Input: part model. Units: mm. Frame: model coordinates. Round coordinates to 2 decimals unless told otherwise and drop trailing zeros. Loops run counter-clockwise (first coordinate to the right, second up) from the corner with the lowest first, then second, coordinate; pieces in that order, holes last. Notation, with made-up numbers: (78, 37.5) - (127, 37.5) arc R5 cw to (127, 44.5) - close; hole circle Ø5 at (-25, 74). An arc over 180 degrees is marked (long way). Use CSV: the item, a comma, the result in double quotes. Start each with the question number.
1. Cut plane A-A (y = 2). Return loops of the section in (x, z), and give its area (3 significant figures).
2. Cut plane B-B (x = 68). Return loops of the section in (y, z).
3. Material intervals for probe 1 along Y at (x, z) = (11.5, 5); probe 2 along X at (y, z) = (3.25, 29.5); probe 3 along Z at (x, y) = (75, -2.5), sorted ascending. Write a range as from..to.
4. Pin query (flat end, axial travel): P1, Ø1, axis at x = 27.5, z = 32.5, coming from the +Y side; P2, Ø5, axis at x = 59.5, y = -1.5, coming from the +Z side; P3, Ø4, axis at y = 2.5, z = 41.5, coming from the +X side; P4, Ø1.5, axis at x = 1.5, z = 30.5, coming from the +Y side. Return the tip coordinate at first contact, or that it passes through.
5. Cut plane C-C (z = 59.5). Return loops of the section in (x, y), and give its area (3 significant figures).
```python
from build123d import *

# Parameters (mm, degrees)
F1_W      = 84
F1_H      = 65
F2_DEPTH  = 3
F3_W      = 3
F3_H      = 3.8
F4_DEPTH  = 5.5
F0_W      = 3
F0_H      = 3.8
F14_DEPTH = 3.5


with BuildPart() as f2:
    # F1 (on Front) → F2 (new body)
    with BuildSketch(Plane.XZ):
        with Locations((42, 32.5)):
            Rectangle(F1_W, F1_H)
    extrude(amount=F2_DEPTH)

    # F3 (on face) → F4 (join)
    with BuildSketch(Plane.XZ):
        with Locations((1.5, 41.1)):
            Rectangle(F3_W, F3_H)
    extrude(amount=-F4_DEPTH)

    # F6: sweep along a path in F0
    with BuildLine(Plane.XZ) as f6_path:
        Line((0, 0), (87, 0))
    # F5 (on face) → F6 (sweep, cut)
    with BuildSketch(Plane(origin=(0, 0, 0), x_dir=(0, -1, 0), z_dir=(-1, 0, 0))):
        Polygon((3, 65), (0, 65), (0, 64), (3, 62), align=None)
        Polygon((0, 1), (0, 0), (3, 0), (3, 3), align=None)
    sweep(path=f6_path.line, mode=Mode.SUBTRACT)

    # F11 (on line) → F12 section 0
    with BuildSketch(Plane(origin=(20, 0, 0), x_dir=(0, -1, 0), z_dir=(-1, 0, 0))):
        with BuildLine():
            Line((3, 30), (3, 35))
            add(Edge.make_bspline(
                [(3, 30), (2.5, 30.5), (2.5, 32.5), (2.5, 34.5), (3, 35)],
                knots=[0, 0, 0, 0, 0.5, 1, 1, 1, 1], degree=3))
        make_face()
    # F9 (on line) → F12 section 1
    with BuildSketch(Plane(origin=(5, 0, 0), x_dir=(0, -1, 0), z_dir=(-1, 0, 0))):
        with BuildLine():
            Line((3, 27.5), (3, 37.5))
            add(Edge.make_bspline(
                [(3, 27.5), (2, 28.5), (-1, 32.5), (2, 36.5), (3, 37.5)],
                knots=[0, 0, 0, 0, 0.5, 1, 1, 1, 1], degree=3))
        make_face()
    loft(mode=Mode.SUBTRACT)

    # F11 (on line) → F13 (revolve, cut)
    with BuildSketch(Plane(origin=(20, 0, 0), x_dir=(0, -1, 0), z_dir=(-1, 0, 0))):
        with BuildLine():
            Line((3, 30), (3, 35))
            add(Edge.make_bspline(
                [(3, 30), (2.5, 30.5), (2.5, 32.5), (2.5, 34.5), (3, 35)],
                knots=[0, 0, 0, 0, 0.5, 1, 1, 1, 1], degree=3))
        make_face()
    revolve(axis=Axis((20, -3, 20), (0, 0, -1)), mode=Mode.SUBTRACT)

    # F0 (on Front) → F14 (join)
    with BuildSketch(Plane.XZ):
        with Locations((1.5, 30.5)):
            Rectangle(F0_W, F0_H)
    extrude(amount=-F14_DEPTH)


solid = f2.part
```
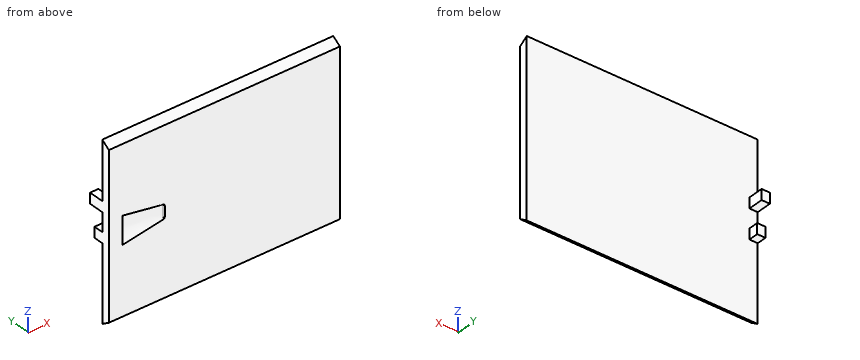
Established:
1,outline,"(0, 28.6) - (3, 28.6) - (3, 32.4) - (0, 32.4) - close; (0, 39.2) - (3, 39.2) - (3, 43) - (0, 43) - close"
1,area,"22.8 mm2"
2,outline,"(-3, 3) - (0, 1) - (0, 64) - (-3, 62) - close"
3,probe 1,"y = -3..0"
3,probe 2,"x = 0..3"
3,probe 3,"z = 2.67..62.33"
4,P1,"stops at y = 0"
4,P2,"stops at z = 64"
4,P3,"stops at x = 3"
4,P4,"stops at y = 3.5"
5,outline,"(0, -3) - (84, -3) - (84, 0) - (0, 0) - close"
5,area,"252 mm2"
